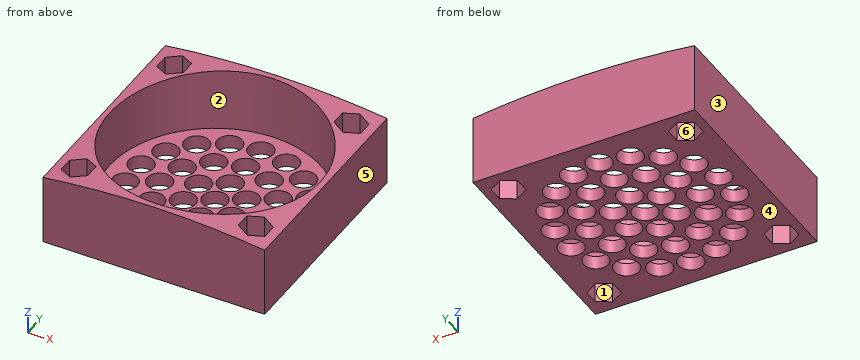
from build123d import *
from build123d import SkipClean  # not in build123d's __all__

# Parameters (mm, degrees)
F0_W     = 40
F0_H     = 40
F1_DEPTH = 13.918
F3_DEPTH = 25
F4_R     = 19
F5_DEPTH = 11.5
F7_DEPTH = 50
F8_R     = 2.25
F9_DEPTH = 25


with BuildPart() as f1:
    # F0 (on Top) → F1 (new body)
    with BuildSketch(Plane.XY):
        Rectangle(F0_W, F0_H)
    extrude(amount=F1_DEPTH)

    # F2 (on face) → F3 (cut)
    with BuildSketch(Plane.XY.offset(13.918)):
        Polygon((-13.6, 17.0143593539), (-16, 18.4), (-18.4, 17.0143593539), (-18.4, 14.2430780618), (-16, 12.8574374158), (-13.6, 14.2430780618), align=None)
        Polygon((13.6, 17.0143593539), (13.6, 14.2430780618), (16, 12.8574374158), (18.4, 14.2430780618), (18.4, 17.0143593539), (16, 18.4), align=None)
        Polygon((-13.6, -17.0143593539), (-13.6, -14.2430780618), (-16, -12.8574374158), (-18.4, -14.2430780618), (-18.4, -17.0143593539), (-16, -18.4), align=None)
        Polygon((18.4, -14.2430780618), (16, -12.8574374158), (13.6, -14.2430780618), (13.6, -17.0143593539), (16, -18.4), (18.4, -17.0143593539), align=None)
    extrude(amount=-F3_DEPTH, mode=Mode.SUBTRACT)

    # F4 (on face) → F5 (cut)
    with BuildSketch(Plane.XY.offset(13.918)):
        Circle(F4_R)
    extrude(amount=-F5_DEPTH, mode=Mode.SUBTRACT)

    # F6 (on face) → F7 (cut)
    with BuildSketch(Plane(origin=(0, 20, 0), x_dir=(-1, 0, 0), z_dir=(0, 1, 0))):
        with BuildLine():
            ThreePointArc((-20, 12.5999645093), (-10.021691693, 13.5881341343), (0, 13.918))
            Line((0, 13.918), (-20, 13.918))
            Line((-20, 13.918), (-20, 12.5999645093))
        make_face()
        with BuildLine():
            ThreePointArc((0, 13.918), (10.021691693, 13.5881341343), (20, 12.5999645093))
            Line((20, 12.5999645093), (20, 13.918))
            Line((20, 13.918), (0, 13.918))
        make_face()
    with SkipClean():  # cleaning this boolean's faces spoils the solid; the shape is the same uncleaned
        extrude(amount=-F7_DEPTH, mode=Mode.SUBTRACT)

    # F8 (on face) → F9 (cut)
    with BuildSketch(Plane(origin=(0, 0, 0), x_dir=(1, 0, 0), z_dir=(0, 0, -1))):
        Circle(F8_R)
        with Locations((0, 5)):
            Circle(F8_R)
        with Locations((-4.3301270189, 2.5)):
            Circle(F8_R)
        with Locations((-4.3301270189, -2.5)):
            Circle(F8_R)
        with Locations((0, -5)):
            Circle(F8_R)
        with Locations((4.3301270189, -2.5)):
            Circle(F8_R)
        with Locations((4.3301270189, 2.5)):
            Circle(F8_R)
        with Locations((0, 10)):
            Circle(F8_R)
        with Locations((0, 15)):
            Circle(F8_R)
        with Locations((-5.1303021499, 14.0953893118)):
            Circle(F8_R)
        with Locations((-9.6418141453, 11.4906666468)):
            Circle(F8_R)
        with Locations((-12.9903810568, 7.5)):
            Circle(F8_R)
        with Locations((-14.7721162952, 2.604722665)):
            Circle(F8_R)
        with Locations((-14.7721162952, -2.604722665)):
            Circle(F8_R)
        with Locations((-12.9903810568, -7.5)):
            Circle(F8_R)
        with Locations((-9.6418141453, -11.4906666468)):
            Circle(F8_R)
        with Locations((-5.1303021499, -14.0953893118)):
            Circle(F8_R)
        with Locations((0, -15)):
            Circle(F8_R)
        with Locations((5.1303021499, -14.0953893118)):
            Circle(F8_R)
        with Locations((9.6418141453, -11.4906666468)):
            Circle(F8_R)
        with Locations((12.9903810568, -7.5)):
            Circle(F8_R)
        with Locations((14.7721162952, -2.604722665)):
            Circle(F8_R)
        with Locations((14.7721162952, 2.604722665)):
            Circle(F8_R)
        with Locations((12.9903810568, 7.5)):
            Circle(F8_R)
        with Locations((9.6418141453, 11.4906666468)):
            Circle(F8_R)
        with Locations((5.1303021499, 14.0953893118)):
            Circle(F8_R)
        with Locations((-5, 8.6602540378)):
            Circle(F8_R)
        with Locations((-8.6602540378, 5)):
            Circle(F8_R)
        with Locations((-10, 0)):
            Circle(F8_R)
        with Locations((-8.6602540378, -5)):
            Circle(F8_R)
        with Locations((-5, -8.6602540378)):
            Circle(F8_R)
        with Locations((0, -10)):
            Circle(F8_R)
        with Locations((5, -8.6602540378)):
            Circle(F8_R)
        with Locations((8.6602540378, -5)):
            Circle(F8_R)
        with Locations((10, 0)):
            Circle(F8_R)
        with Locations((8.6602540378, 5)):
            Circle(F8_R)
        with Locations((5, 8.6602540378)):
            Circle(F8_R)
    with SkipClean():  # cleaning this boolean's faces spoils the solid; the shape is the same uncleaned
        extrude(amount=-F9_DEPTH, mode=Mode.SUBTRACT)


solid = f1.part
Can you work these out from the model? Positions are in its coordinate system, mm. Face numbers are marked on the shaded views. A direction names the side the tool comes from. Give positions to 0.01 mm unless a question says otherwise; leave off trailing zeros. Loops run counter-clockwise (first coordinate to the right, second up) from the corner with the lowest first, then second, coordinate; pieces in that order, holes last. Notation, with made-up numbers: M 18,8.5 L 22,8.5 A22 cw 22,45.5 Z; hole C 1.25,17.25 d11. An arc over 180 degrees is marked long. One line per item, written item: value. Start each with the question number.
1) On a 3-axis mill with a long thin cutter (end or side, diameter ignored), from which of +Z, -Z, +X, -X, +Y, -Y can I reach the whole of each face in a straight line? I mean the marked faces 5 and 6. Say none if no direction works.
2) If we section it at C-C, the plane y = -15: Write out the boundary of the cut face in (x, z).
3) I'm going to push flat-ended pins straight in: pin 1 (3 mm diameter, centred on x = 10, y = 6.5, fed in from +Z); pin 2 (12 mm diameter, centred on x = 1.5, y = 9.5, fed in from -Z). Where does each tip first touch, or does it pass through?
4) If I drill on line 1 (X direction, y = 0, z = 10); line 2 (X direction, y = 13, z = 10.25), over which ranges is the centre line in solid material (lowest first)? Write a range as [from, to].
5) If we section it at B-B, the plane x = 10: Write out the boundary of the cut face in (y, z), and give its area (3 significant figures).
6) Thinking about a two-plate mould opening in X: for the marked faces 1, 2, 3 and 4, which applies, +X half, -X half, draft (parallel to the pull), parting line (faces both ways), or undercut?
7) If we section it at A-A, the plane z = 10: Give the number of separate pieces and of enclosed holes in the cut face, and give its area (3 significant figures).
Completed:
1. face 5: +Z, -Z, +X, +Y, -Y
1. face 6: +Z, -Z
2. outline: M -20,0 L -18.4,0 L -18.4,12.8 A152.4 ccw -20,12.6 Z; M -13.6,0 L -7.19,0 L -7.19,2.42 L -11.66,2.42 L -11.66,13.47 A152.4 ccw -13.6,13.31 Z; M -3.07,0 L -2.25,0 L -2.25,2.42 L -3.07,2.42 Z; M 2.25,0 L 3.07,0 L 3.07,2.42 L 2.25,2.42 Z; M 7.19,0 L 13.6,0 L 13.6,13.31 A152.4 ccw 11.66,13.47 L 11.66,2.42 L 7.19,2.42 Z; M 18.4,0 L 20,0 L 20,12.6 A152.4 ccw 18.4,12.8 Z
3. pin 1: stops at z = 2.42
3. pin 2: stops at z = 0
4. line 1: x = [-20, -19], [19, 20]
4. line 2: x = [-20, -16.25], [-15.75, -13.86], [13.86, 15.75], [16.25, 20]
5. outline: M -20,0 L -13.71,0 L -13.71,2.42 L -16.16,2.42 L -16.16,13.59 L -20,13.59 Z; M -9.27,0 L -6.81,0 L -6.81,2.42 L -9.27,2.42 Z; M -3.19,0 L -2.25,0 L -2.25,2.42 L -3.19,2.42 Z; M 2.25,0 L 3.19,0 L 3.19,2.42 L 2.25,2.42 Z; M 6.81,0 L 9.27,0 L 9.27,2.42 L 6.81,2.42 Z; M 13.71,0 L 20,0 L 20,13.59 L 16.16,13.59 L 16.16,2.42 L 13.71,2.42 Z
5. area: 133 mm^2
6. face 1: undercut
6. face 2: undercut
6. face 3: -X half
6. face 4: draft
7. separate pieces: 1
7. enclosed holes: 5
7. area: 386 mm^2
